Design review of the part shown in the three views and the two pictorial views. Dimensions are in mm from the part's minimum x, y and z. A direction names the side the tool comes from. Give positions to 0.01 mm unless a question says otherwise; leave off trailing zeros. Loops run counter-clockwise (first coordinate to the right, second up) from the corner with the lowest first, then second, coordinate; pieces in that order, holes last. Notation, with made-up numbers: (68.5, -8) - (74.5, -8) arc R29 ccw to (74.5, 22) - close; hole circle Ø2 at (89, 14). An arc over 180 degrees is marked (long way). Use CSV: the item, a comma, the result in double quotes. Start each with the question number.
1. Wall thickness on line 1 (Z direction, x = 6, y = 1.5); line 2 (X direction, y = 2.25, z = 11); line 3 (X direction, y = 2, z = 6): over which ranges is each line inside the solid? List them lowest first.
2. For the marked faces 1 and 2, list the 3-axis set-ups (+Z, -Z, +X, -X, +Y, -Y) from which the entire face can be reached by the end or side of a thin tool; tool diameter is ignored.
3. Take a section at A-A on y = 4.5. Give the boundary of the cut face in (x, z).
4. For pin 1 (4 mm diameter, centred on y = 7, z = 2.5, fed in from -X); pin 2 (4 mm diameter, centred on y = 1.5, z = 7.5, fed in from -X); pin 3 (5 mm diameter, centred on y = 3.5, z = 8.5, fed in from +X), all flat-tipped, find the tip position at first contact; note any pin that passes through.
5. Take a section at C-C on z = 3.25. Give the boundary of the cut face in (x, y).
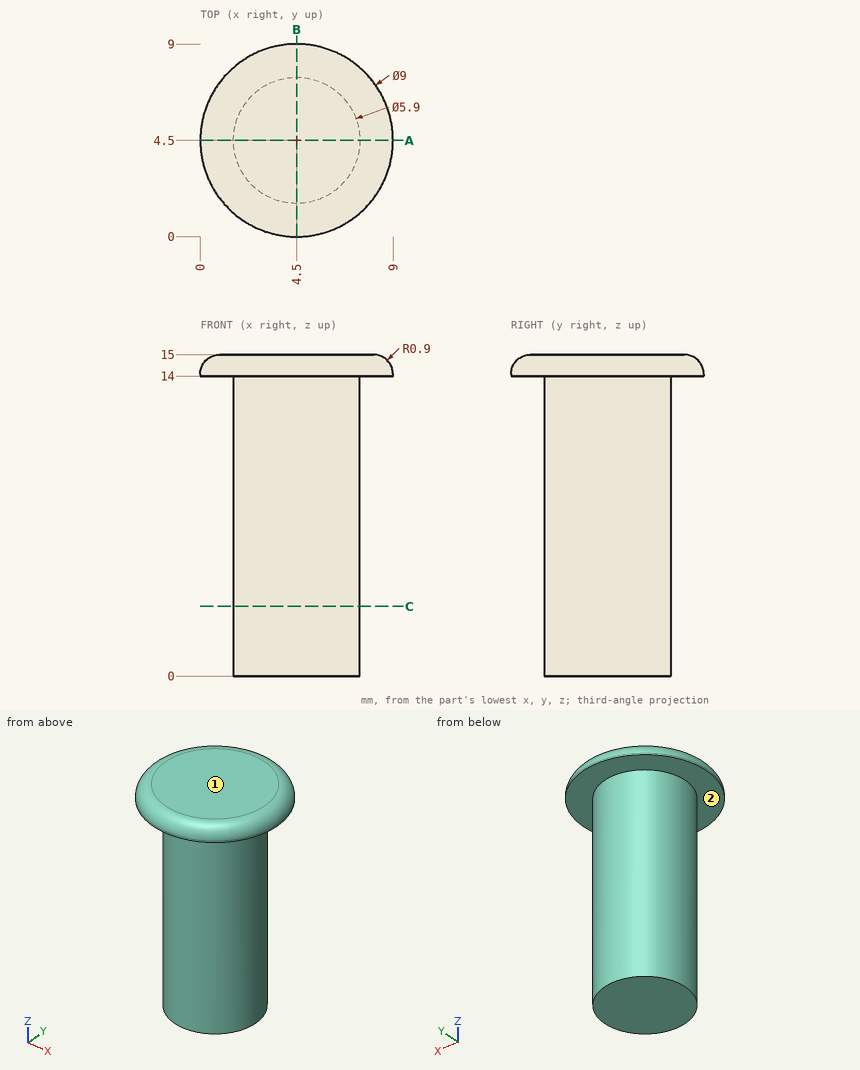
Check result:
1,line 1,"z = 14 to 15"
1,line 2,"x = 2.59 to 6.41"
1,line 3,"x = 2.93 to 6.07"
2,face 1,"+Z, +X, -X, +Y, -Y"
2,face 2,"-Z"
3,outline,"(0, 14) - (1.55, 14) - (1.55, 0) - (7.45, 0) - (7.45, 14) - (9, 14) - (9, 14.1) arc R0.9 ccw to (8.1, 15) - (0.9, 15) arc R0.9 ccw to (0, 14.1) - close"
4,pin 1,"stops at x = 1.59"
4,pin 2,"stops at x = 1.72"
4,pin 3,"stops at x = 7.45"
5,outline,"circle Ø5.9 at (4.5, 4.5)"
